Model file for the job. Use its own axes, mm. A direction names the side the tool comes from. Give positions to 0.01 mm unless a question says otherwise; leave off trailing zeros. Write each loop counter-clockwise with the first axis right and the second up, starting at its lowest first coordinate (ties: lowest second). Pieces come first, ordered by that corner, then holes. Notation, with made-up numbers: (17, 60.25) - (54, 60.25) arc R13 ccw to (54, 67.25) - close; hole circle Ø9 at (43, 48). An arc over 180 degrees is marked (long way). Use a Markdown table: item, result. Add a question column.
```python
from build123d import *

# Parameters (mm, degrees)
SKETCH1_W                = 24.5
SKETCH1_H                = 76
BASE_FLANGE1_DEPTH       = 0.86
EDGE_FLANGE1_DEPTH       = 76
EDGE_FLANGE4_DEPTH       = 76
EDGE_FLANGE5_DEPTH       = 34.909250773
EDGE_FLANGE6_DEPTH       = 34.938
EDGE_FLANGE7_DEPTH       = 77.5
SKETCH40_W               = 5.238
SKETCH40_H               = 18.938
CUT_EXTRUDE1_DEPTH       = 10
SKETCH41_W               = 5.238
SKETCH41_H               = 18.909250773
CUT_EXTRUDE2_DEPTH       = 10
FILLET1_R                = 3
FILLET2_R                = 3
EDGE_FLANGE9_START       = -38
EDGE_FLANGE9_DEPTH       = 77.5
EDGE_FLANGE9_2_DEPTH     = 77.5
M3_CLEARANCE_HOLE2_D     = 3.4
M3_CLEARANCE_HOLE2_DEPTH = 28.71
M3_CLEARANCE_HOLE2_TIP   = 1.021463052
FILLET4_R                = 6
SKETCH51_W               = 26.616
SKETCH51_H               = 5.735679753
CUT_EXTRUDE4_DEPTH       = 10
FILLET5_R                = 4
HEX_PATTERN_DEPTH        = 74.517332053


# Read off the part's stored shape, not the designer's step: Edge-Flange9
# Sheet-metal steps are written as plain solids
with BuildPart() as part:
    # Sketch1 → Base-Flange1 (new body)
    with BuildSketch(Plane(origin=(0, 0, 0), x_dir=(1, 0, 0), z_dir=(0, 1, 0))):
        Rectangle(SKETCH1_W, SKETCH1_H)
    extrude(amount=-BASE_FLANGE1_DEPTH)

    # Edge-Flange1 section (across the edge) → Edge-Flange1 (add)
    with BuildSketch(Plane(origin=(14.762, 0, 38), x_dir=(-1, 0, 0), z_dir=(0, 0, -1))):
        with BuildLine():
            Line((-0.86, 0.762), (-0.86, 52.3))
            Line((-0.86, 52.3), (0, 52.3))
            Line((0, 52.3), (0, 0.762))
            ThreePointArc((0, 0.762), (0.223184633, 0.223184633), (0.762, 0))
            Line((0.762, 0), (2.512, 0))
            Line((2.512, 0), (2.512, -0.86))
            Line((2.512, -0.86), (0.762, -0.86))
            ThreePointArc((0.762, -0.86), (-0.384927199, -0.384927199), (-0.86, 0.762))
        make_face()
    extrude(amount=EDGE_FLANGE1_DEPTH)

    # Edge-Flange4 section (across the edge) → Edge-Flange4 (add)
    with BuildSketch(Plane(origin=(-14.762, 0, -38), x_dir=(1, 0, 0), z_dir=(0, 0, 1))):
        with BuildLine():
            Line((-0.86, 0.762), (-0.86, 35.7))
            Line((-0.86, 35.7), (0, 35.7))
            Line((0, 35.7), (0, 0.762))
            ThreePointArc((0, 0.762), (0.223184633, 0.223184633), (0.762, 0))
            Line((0.762, 0), (2.512, 0))
            Line((2.512, 0), (2.512, -0.86))
            Line((2.512, -0.86), (0.762, -0.86))
            ThreePointArc((0.762, -0.86), (-0.384927199, -0.384927199), (-0.86, 0.762))
        make_face()
    extrude(amount=EDGE_FLANGE4_DEPTH)

    # Edge-Flange5 section (across the edge) → Edge-Flange5 (add)
    with BuildSketch(Plane(origin=(14.762, 0.762, 40.262), x_dir=(0, 0, -1), z_dir=(0, 1, 0))):
        with BuildLine():
            Line((-0.86, 0.762), (-0.86, 14))
            Line((-0.86, 14), (0, 14))
            Line((0, 14), (0, 0.762))
            ThreePointArc((0, 0.762), (0.223184633, 0.223184633), (0.762, 0))
            Line((0.762, 0), (2.262, 0))
            Line((2.262, 0), (2.262, -0.86))
            Line((2.262, -0.86), (0.762, -0.86))
            ThreePointArc((0.762, -0.86), (-0.384927199, -0.384927199), (-0.86, 0.762))
        make_face()
    extrude(amount=EDGE_FLANGE5_DEPTH)

    # Edge-Flange6 section (across the edge) → Edge-Flange6 (add)
    with BuildSketch(Plane(origin=(-14.762, 35.7, 40.262), x_dir=(0, 0, -1), z_dir=(0, -1, 0))):
        with BuildLine():
            Line((-0.86, 0.762), (-0.86, 14))
            Line((-0.86, 14), (0, 14))
            Line((0, 14), (0, 0.762))
            ThreePointArc((0, 0.762), (0.223184633, 0.223184633), (0.762, 0))
            Line((0.762, 0), (2.262, 0))
            Line((2.262, 0), (2.262, -0.86))
            Line((2.262, -0.86), (0.762, -0.86))
            ThreePointArc((0.762, -0.86), (-0.384927199, -0.384927199), (-0.86, 0.762))
        make_face()
    extrude(amount=EDGE_FLANGE6_DEPTH)

    # Edge-Flange7 section (across the edge) → Edge-Flange7 (add)
    with BuildSketch(Plane(origin=(-14.762, 36.462, -38), x_dir=(0, -1, 0), z_dir=(0, 0, 1))):
        with BuildLine():
            Line((-0.86, 0.762), (-0.86, 29))
            Line((-0.86, 29), (0, 29))
            Line((0, 29), (0, 0.762))
            ThreePointArc((0, 0.762), (0.223184633, 0.223184633), (0.762, 0))
            Line((0.762, 0), (0.762, -0.86))
            ThreePointArc((0.762, -0.86), (-0.384927199, -0.384927199), (-0.86, 0.762))
        make_face()
    extrude(amount=EDGE_FLANGE7_DEPTH)

    # Sketch40 → Cut-Extrude1 (cut)
    with BuildSketch(Plane.XY.offset(41.122)):
        with Locations((-3.381, 18.231)):
            Rectangle(SKETCH40_W, SKETCH40_H)
    extrude(amount=-CUT_EXTRUDE1_DEPTH, mode=Mode.SUBTRACT)

    # Sketch41 → Cut-Extrude2 (cut)
    with BuildSketch(Plane.XY.offset(41.122)):
        with Locations((3.381, 18.216625386)):
            Rectangle(SKETCH41_W, SKETCH41_H)
    extrude(amount=-CUT_EXTRUDE2_DEPTH, mode=Mode.SUBTRACT)

    # Fillet1
    fillet1_edges = [part.edges().sort_by_distance(p)[0] for p in [
        (-0.762, 8.762, 40.692),
        (-0.762, 27.7, 40.692),
        (0.762, 8.762, 40.692),
        (0.762, 27.671250773, 40.692),
    ]]
    fillet(fillet1_edges, radius=FILLET1_R)

    # Fillet2
    fillet2_edges = [part.edges().sort_by_distance(p)[0] for p in [
        (-6, 8.762, 40.692),
        (6, 8.762, 40.692),
        (6, 27.671250773, 40.692),
        (-6, 27.7, 40.692),
    ]]
    fillet(fillet2_edges, radius=FILLET2_R)

    # Edge-Flange9 outline → Edge-Flange9 (cut)
    with BuildSketch(Plane.XY.offset(EDGE_FLANGE9_START)):
        with BuildLine():
            Line((14.238, 37.322), (14.047865915, 37.322))
            ThreePointArc((14.047865915, 37.322), (13.451140707, 36.693523823), (12.616, 36.462))
            Line((12.616, 36.462), (14.238, 36.462))
            Line((14.238, 36.462), (14.238, 37.322))
        make_face()
    extrude(amount=EDGE_FLANGE9_DEPTH, mode=Mode.SUBTRACT)

    # Edge-Flange9 2 outline → Edge-Flange9 2 (add)
    with BuildSketch(Plane.XY.offset(EDGE_FLANGE9_START)):
        with BuildLine():
            ThreePointArc((14.047865915, 37.322), (14.189748791, 37.691318523), (14.238, 38.084))
            Line((14.238, 38.084), (14.238, 52.322))
            Line((14.238, 52.322), (13.378, 52.322))
            Line((13.378, 52.322), (13.378, 38.084))
            ThreePointArc((13.378, 38.084), (13.154815367, 37.545184633), (12.616, 37.322))
            Line((12.616, 37.322), (14.047865915, 37.322))
        make_face()
    extrude(amount=EDGE_FLANGE9_2_DEPTH)

    # M3 Clearance Hole2
    with Locations(Plane.ZY.offset(-13.378)):
        with Locations((-18, 44.822), (19.5, 44.822)):
            Hole(M3_CLEARANCE_HOLE2_D / 2, depth=M3_CLEARANCE_HOLE2_DEPTH)
            with Locations((0, 0, -(M3_CLEARANCE_HOLE2_DEPTH + M3_CLEARANCE_HOLE2_TIP / 2))):  # 118° drill point
                Cone(0, M3_CLEARANCE_HOLE2_D / 2, M3_CLEARANCE_HOLE2_TIP, mode=Mode.SUBTRACT)

    # Fillet4
    fillet4_edges = [part.edges().sort_by_distance(p)[0] for p in [
        (13.808, 52.322, 39.5),
        (13.808, 52.322, -38),
    ]]
    fillet(fillet4_edges, radius=FILLET4_R)

    # Sketch51 → Cut-Extrude4 (cut)
    with BuildSketch(Plane(origin=(0, 37.322, 0), x_dir=(1, 0, 0), z_dir=(0, 1, 0))):
        with Locations((-0.692, 35.132160124)):
            Rectangle(SKETCH51_W, SKETCH51_H)
    extrude(amount=-CUT_EXTRUDE4_DEPTH, mode=Mode.SUBTRACT)

    # Fillet5
    fillet5_edges = [part.edges().sort_by_distance(p)[0] for p in [
        (-14, 36.892, -32.264320247),
        (12.616, 36.892, -32.264320247),
    ]]
    fillet(fillet5_edges, radius=FILLET5_R)

    # Sketch52 → Hex Pattern (cut, through all)
    with BuildSketch(Plane.ZY.offset(15.622)):
        Polygon((13.740381057, 30.731), (34.5, 30.731), (34.5, 20.731), (19.513883749, 20.731), align=None)
        Polygon((15.18375673, 18.231), (7.966878365, 30.731), (-6.466878365, 30.731), (-13.68375673, 18.231), (-6.466878365, 5.731), (7.966878365, 5.731), align=None)
        Polygon((-18.013883749, 20.731), (-12.240381057, 30.731), (-33, 30.731), (-33, 20.731), align=None)
        Polygon((-18.013883749, 15.731), (-12.240381057, 5.731), (-33, 5.731), (-33, 15.731), align=None)
        Polygon((19.513883749, 15.731), (13.740381057, 5.731), (34.5, 5.731), (34.5, 15.731), align=None)
    extrude(amount=-HEX_PATTERN_DEPTH, mode=Mode.SUBTRACT)


solid = part.part
```
(1) Probe probe 1 along Y at (x, z) = (7, 4.5); probe 2 along X at (y, z) = (22, 14); probe 3 along Y at (x, z) = (13.7, -18). List the from-to ranges inside material, lowest first. Write a range as [from, to].
(2) Two-plate mould, pull along X, no slides. Class faces 1 (the cylindrical face through (-1.49, 7.72, 40.69)), 2 (the cylindrical face through (-15.159, 18.476, 40.634)), 3 (the flat face through (0, 0, -1)), 4 (the cylindrical face through (13.814, 46.508, 19.721)): +X half, -X half, draft (parallel to the pull), parting line (faces both ways), or undercut.
(3) Band-saw the part on A-A (z = -5.5). Write the cut outline in (x, y).
(4) Band-saw the part on B-B (x = 11.5). Write the cut outline in (y, z), then the cut area to 3 significant figures.
(5) Band-saw the part on D-D (z = 30). Give the number of separate pieces and of enclosed holes in the cut face, then the cut area to 3 significant figures.
(6) Band-saw the part on C-C (x = -2). Write the cut outline in (y, z).
(7) Flat gauge pins, fed straight in: pin 1 (8.5 mm diameter, centred on x = 6, z = -6, fed in from +Y); pin 2 (0.9 mm diameter, centred on x = -15, y = 12.5, fed in from +Z); pin 3 (0.7 mm diameter, centred on x = 15, z = 10, fed in from +Y). Where does each tip first touch, or does it go through?
(8) Which spindle directions (+Z, -Z, +X, -X, +Y, -Y) get a long thin tool onto all of the face, cutting with end or side? Do faces 5 (the flat face through (-9, 18, 40.262)), 6 (the flat face through (13.378, 45, 0)), 7 (the flat face through (15.186, 10.801, -15.168)). Say none if no direction does.
Model answer:
| question | item | result |
|---|---|---|
| 1 | probe 1 | y = [-0.86, 0], [36.46, 37.32] |
| 1 | probe 2 | x = [-15.62, -14.76], [14.76, 15.62] |
| 1 | probe 3 | y = [-0.86, 0], [36.88, 43.12], [46.52, 52.32] |
| 2 | face 1 | undercut |
| 2 | face 2 | -X half |
| 2 | face 3 | undercut |
| 2 | face 4 | draft |
| 3 | outline | (-15.62, 0.76) arc R1.62 ccw to (-14, -0.86) - (14, -0.86) arc R1.62 ccw to (15.62, 0.76) - (15.62, 5.73) - (14.76, 5.73) - (14.76, 0.76) arc R0.76 cw to (14, 0) - (-14, 0) arc R0.76 cw to (-14.76, 0.76) - (-14.76, 5.73) - (-15.62, 5.73) - close; (-15.62, 30.73) - (-14.76, 30.73) - (-14.76, 35.7) arc R0.76 cw to (-14, 36.46) - (12.62, 36.46) arc R1.62 ccw to (14.24, 38.08) - (14.24, 52.32) - (13.38, 52.32) - (13.38, 38.08) arc R0.76 cw to (12.62, 37.32) - (-14, 37.32) arc R1.62 ccw to (-15.62, 35.7) - close; (14.76, 30.73) - (15.62, 30.73) - (15.62, 52.3) - (14.76, 52.3) - close |
| 4 | outline | (-0.86, -38) - (0, -38) - (0, 38) - (-0.86, 38) - close; (0.76, 40.26) - (35.67, 40.26) - (35.67, 41.12) - (0.76, 41.12) - close; (36.46, -33.49) - (37.32, -33.49) - (37.32, 39.5) - (36.46, 39.5) - close |
| 4 | area | 158 mm^2 |
| 5 | separate pieces | 5 |
| 5 | enclosed holes | 0 |
| 5 | area | 106 mm^2 |
| 6 | outline | (-0.86, -38) - (0, -38) - (0, 38) - (-0.86, 38) - close; (0.76, 40.26) - (8.19, 40.26) - (8.19, 41.12) - (0.76, 41.12) - close; (28.27, 40.26) - (35.7, 40.26) - (35.7, 41.12) - (28.27, 41.12) - close; (36.46, -32.26) - (37.32, -32.26) - (37.32, 39.5) - (36.46, 39.5) - close |
| 7 | pin 1 | stops at y = 37.32 |
| 7 | pin 2 | stops at z = 41.03 |
| 7 | pin 3 | stops at y = 52.3 |
| 8 | face 5 | -Z, +Y, -Y |
| 8 | face 6 | +Z, -Z, -X, +Y |
| 8 | face 7 | +X, -X |
